from build123d import *

# Parameters (mm, degrees)
BOSS_EXTRUDE1_DEPTH                             = 12
CBORE_FOR_M5_SOCKET_HEAD_CAP_SCREW1_D           = 5.5
CBORE_FOR_M5_SOCKET_HEAD_CAP_SCREW1_CBORE_D     = 10
CBORE_FOR_M5_SOCKET_HEAD_CAP_SCREW1_CBORE_DEPTH = 5
M5X0_8_TAPPED_HOLE1_D                           = 4.2
M5X0_8_TAPPED_HOLE1_DEPTH                       = 14
M5X0_8_TAPPED_HOLE1_TIP                         = 1.2618073


with BuildPart() as part:
    # Sketch1 → Boss-Extrude1 (new body)
    with BuildSketch(Plane.XY):
        Polygon((-47.5, 20), (-52.5, 15), (-52.5, 0), (52.5, 0), (52.5, 15), (47.5, 20), align=None)
    extrude(amount=BOSS_EXTRUDE1_DEPTH)

    # CBORE for M5 Socket Head Cap Screw1 (through all)
    with Locations(Plane.XY.offset(12)):
        with Locations((-17, 12)):
            CounterBoreHole(CBORE_FOR_M5_SOCKET_HEAD_CAP_SCREW1_D / 2, CBORE_FOR_M5_SOCKET_HEAD_CAP_SCREW1_CBORE_D / 2, CBORE_FOR_M5_SOCKET_HEAD_CAP_SCREW1_CBORE_DEPTH)

    # M5x0.8 Tapped Hole1
    with Locations(Plane.XZ):
        with Locations((-37.5, 6), (37.5, 6)):
            Hole(M5X0_8_TAPPED_HOLE1_D / 2, depth=M5X0_8_TAPPED_HOLE1_DEPTH)
            with Locations((0, 0, -(M5X0_8_TAPPED_HOLE1_DEPTH + M5X0_8_TAPPED_HOLE1_TIP / 2))):  # 118° drill point
                Cone(0, M5X0_8_TAPPED_HOLE1_D / 2, M5X0_8_TAPPED_HOLE1_TIP, mode=Mode.SUBTRACT)


solid = part.part
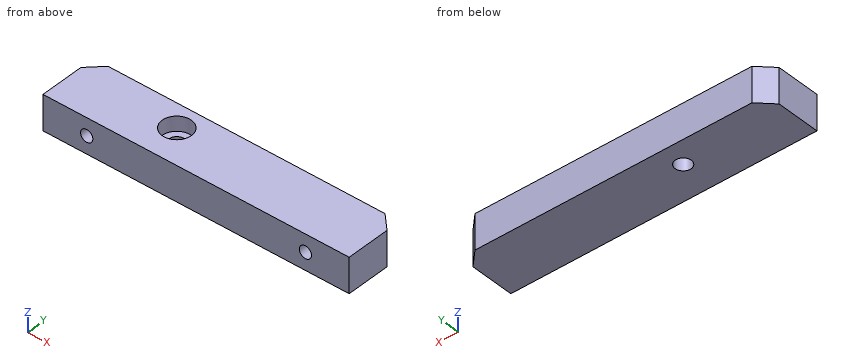
Geometry: final body of the model. Coordinates: model frame, mm. Give positions to 0.01 mm unless a question says otherwise; leave off trailing zeros. Write each loop counter-clockwise with the first axis right and the second up, starting at its lowest first coordinate (ties: lowest second). Pieces come first, ordered by that corner, then holes. Notation, with made-up numbers: (71.25, 55) -> (119.25, 55) arc R22 cw to (119.25, 63) -> close; hole circle Ø4 at (45, 50). An arc over 180 degrees is marked (long way). Answer in a Markdown table with one row per item.
(1) Section query A-A on z = 10.5. Return loops of the section in (x, y), then the cut area to 3 significant figures.
Answers below:
| item | result |
|---|---|
| outline | (-52.5, 0) -> (52.5, 0) -> (52.5, 15) -> (47.5, 20) -> (-47.5, 20) -> (-52.5, 15) -> close; hole circle Ø10 at (-17, 12) |
| area | 2,000 mm^2 |
(2) Section query B-B on y = 10.75. Return loops of the section in (x, z).
Answers below:
| item | result |
|---|---|
| outline | (-52.5, 0) -> (-19.45, 0) -> (-19.45, 7) -> (-21.84, 7) -> (-21.84, 12) -> (-52.5, 12) -> close; (-14.55, 0) -> (52.5, 0) -> (52.5, 12) -> (-12.16, 12) -> (-12.16, 7) -> (-14.55, 7) -> close; hole circle Ø4.2 at (-37.5, 6); hole circle Ø4.2 at (37.5, 6) |
(3) Pin query (flat end, axial travel): pin 1 (4 mm diameter, centred on x = -37.5, z = 6, fed in from -Y); pin 2 (2 mm diameter, centred on y = 17, z = 3, fed in from +X). Return the tip coordinate at first contact, or that it passes through.
Answers below:
| item | result |
|---|---|
| pin 1 | y = 14.06 |
| pin 2 | x = 51.5 |
(4) Ray query, line 1 along X through (y, z) = (6, 6); line 2 along Y through (x, z) = (-17, 3.5); line 3 along Z through (x, y) = (-37.5, 10). Return the intervals inside material, ascending. Write a range as [from, to].
Answers below:
| item | result |
|---|---|
| line 1 | [-52.5, -39.6], [-35.4, 35.4], [39.6, 52.5] |
| line 2 | [0, 9.25], [14.75, 20] |
| line 3 | [0, 3.9], [8.1, 12] |
(5) Section query D-D on y = 2.5. Return loops of the section in (x, z), then the cut area to 3 significant figures.
Answers below:
| item | result |
|---|---|
| outline | (-52.5, 0) -> (52.5, 0) -> (52.5, 12) -> (-52.5, 12) -> close; hole circle Ø4.2 at (-37.5, 6); hole circle Ø4.2 at (37.5, 6) |
| area | 1,230 mm^2 |
(6) Section query C-C on x = -17. Return loops of the section in (y, z).
Answers below:
| item | result |
|---|---|
| outline | (0, 0) -> (9.25, 0) -> (9.25, 7) -> (7, 7) -> (7, 12) -> (0, 12) -> close; (14.75, 0) -> (20, 0) -> (20, 12) -> (17, 12) -> (17, 7) -> (14.75, 7) -> close |
